Build history of the part. All positions in model axes, mm. A direction names the side the tool comes from. Round coordinates to 2 decimals unless told otherwise and drop trailing zeros. Loops run counter-clockwise (first coordinate to the right, second up) from the corner with the lowest first, then second, coordinate; pieces in that order, holes last. Notation, with made-up numbers: (15, 67) -> (73, 67) arc R27 ccw to (73, 100) -> close; hole circle Ø4 at (23, 15). An arc over 180 degrees is marked (long way). Put each result on its own line as item: value. Start each with the question number.
Item 1: Cut at A-A, the plane z = 0. List the corners of the cut face in (x, y) (3 decimals), plus the area to 3 significant figures.
Item 2: Cut at B-B, the plane x = 27.5. List the corners of the cut face in (y, z) (3 decimals), plus the area to 4 significant figures.
Item 3: Cut at D-D, the plane z = 2.75. List the corners of the cut face in (x, y).
Item 4: Tool access for faces 5 (the flat face through (2, 11, 4.5)), 6 (the flat face through (18, 3, 0)): list every direction of +Z, -Z, +X, -X, +Y, -Y with a clear straight run to the whole face (end or side of a thin tool).
Item 5: Drill centre lines: probe 1 along Y at (x, z) = (2.45, 0) (3 decimals); probe 2 along X at (y, z) = (7, -1). Where is each one in solid material? Low to high. Write a range as [from, to].
Item 6: Flat gauge pins, fed straight in: pin 1 Ø3.5 at (y, z) = (27.5, 0) entering from -X; pin 2 Ø1.5 at (y, z) = (9.5, -3) entering from +X; pin 3 Ø4.5 at (x, z) = (22, 0) entering from +Y. Where does each tip first touch, or does it go through?
Item 7: Pull direction Y, two halves, no side cores. Call faces 1 (the flat face through (1, 32, 0)), 2 (the cylindrical face through (1.48, 29.51, -0.26)), 3 (the flat face through (3, 18, 0)), 4 (the cylindrical face through (0.57, 0.6, 0.06)): +Y half, -Y half, draft (parallel to the pull), parting line (faces both ways), or undercut.
```python
from build123d import *

# Parameters (mm, degrees)
SKETCH_1_W          = 3
SKETCH_1_H          = 29
SKETCH_1_W_2        = 32
SKETCH_1_H_2        = 3
EXTRUDE_1_DEPTH     = 4.5
SKETCH_3_R          = 2.025
CUT_EXTRUDE_1_DEPTH = 9
SKETCH_4_R          = 2.025
CUT_EXTRUDE_2_DEPTH = 9
FILLET_1_R          = 2


with BuildPart() as part:
    # 草图1 → 凸台-拉伸1 (new body, symmetric)
    with BuildSketch(Plane.XY):
        with Locations((1.5, 17.5)):
            Rectangle(SKETCH_1_W, SKETCH_1_H)
        with Locations((16, 1.5)):
            Rectangle(SKETCH_1_W_2, SKETCH_1_H_2)
    extrude(amount=EXTRUDE_1_DEPTH, both=True)

    # 草图3 → 切除-拉伸1 (cut)
    with BuildSketch(Plane.XZ):
        with Locations((13.5, 0)):
            Circle(SKETCH_3_R)
        with Locations((27.5, 0)):
            Circle(SKETCH_3_R)
    extrude(amount=-CUT_EXTRUDE_1_DEPTH, mode=Mode.SUBTRACT)

    # 草图4 → 切除-拉伸2 (cut)
    with BuildSketch(Plane.ZY):
        with Locations((0, 27.5)):
            Circle(SKETCH_4_R)
        with Locations((0, 13.5)):
            Circle(SKETCH_4_R)
    extrude(amount=-CUT_EXTRUDE_2_DEPTH, mode=Mode.SUBTRACT)

    # 圆角1
    fillet_1_edges = [part.edges().sort_by_distance(p)[0] for p in [
        (3, 3, 0),
        (0, 0, 0),
    ]]
    fillet(fillet_1_edges, radius=FILLET_1_R)


solid = part.part
```
Reply:
1. outline: (0, 2) arc R2 ccw to (2, 0) -> (11.475, 0) -> (11.475, 3) -> (5, 3) arc R2 cw to (3, 5) -> (3, 11.475) -> (0, 11.475) -> close; (0, 15.525) -> (3, 15.525) -> (3, 25.475) -> (0, 25.475) -> close; (0, 29.525) -> (3, 29.525) -> (3, 32) -> (0, 32) -> close; (15.525, 0) -> (25.475, 0) -> (25.475, 3) -> (15.525, 3) -> close; (29.525, 0) -> (32, 0) -> (32, 3) -> (29.525, 3) -> close
1. area: 134 mm^2
2. outline: (0, -4.5) -> (3, -4.5) -> (3, -2.025) -> (0, -2.025) -> close; (0, 2.025) -> (3, 2.025) -> (3, 4.5) -> (0, 4.5) -> close
2. area: 14.85 mm^2
3. outline: (0, 2) arc R2 ccw to (2, 0) -> (32, 0) -> (32, 3) -> (5, 3) arc R2 cw to (3, 5) -> (3, 32) -> (0, 32) -> close
4. face 5: +Z, +X, -X, +Y, -Y
4. face 6: +Z, -Z, +X, +Y
5. probe 1: y = [0, 11.475], [15.525, 25.475], [29.525, 32]
5. probe 2: x = [0, 3]
6. pin 1: passes through
6. pin 2: stops at x = 3
6. pin 3: stops at y = 3
7. face 1: +Y half
7. face 2: undercut
7. face 3: draft
7. face 4: -Y half
